Read the model definition and answer for the solid it produces. Units are mm, in the model's axes. A direction names the side the tool comes from. Give positions to 0.01 mm unless a question says otherwise; leave off trailing zeros. Order: outer loops, then holes, each group sorted by start corner. A loop starts at its lowest first (then second) coordinate and runs counter-clockwise, first axis right, second up.
Item 1: Which of the six approach directions +Z, -Z, +X, -X, +Y, -Y give full straight-line access (tool end or side, diameter ignored) to faces 5 (the face through (20, 21, -20)), 6 (the face through (35, 0, -20)), 7 (the face through (58, 21, -30))?
Item 2: The mould has two halves that part along X. Classify faces 1 (the face through (20, 30, -30)), 2 (the face through (0, 15, -25)), 3 (the face through (70, 5, -20)), 4 (the face through (5, 40, -30)): +X half, -X half, draft (parallel to the pull), parting line (faces both ways), or undercut.
Item 3: A cutting plane is placed at C-C (x = 20). Write down the section's boundary in (y, z), plus the area to 3 significant figures.
Item 4: Given pin 1 Ø6 at (x, y) = (44, 25.5) entering from +Z; pin 2 Ø16 at (x, y) = (61, 21.5) entering from +Z; pin 3 Ø9 at (x, y) = (22.5, 21.5) entering from +Z; pin 4 Ø3 at (y, z) = (27.5, -18) entering from -X, each flat-ended and moving along its own axis, determine where each tip first touches the part or whether it passes through.
Item 5: A cutting plane is placed at D-D (x = 61). Write down the section's boundary in (y, z).
Item 6: A cutting plane is placed at B-B (z = -36.5). Write down the section's boundary in (x, y), plus the area to 3 significant figures.
Item 7: Find the intervals of material crossed by line 1 along Z through (x, y) = (60, 11); line 2 along Y through (x, z) = (18, -14); line 3 along Z through (x, y) = (12, 17.5), in increasing order.
Autodesk Inventor part; units mm, degrees
ref_plane "YZ Plane" through (0, 0, 0) normal (1, 0, 0) x (0, 1, 0)
ref_plane "XZ Plane" through (0, 0, 0) normal (0, 1, 0) x (-1, 0, 0)
ref_plane "XY Plane" through (0, 0, 0) normal (0, 0, 1) x (1, 0, 0)
sketch "草圖1" plane through (0, 0, 0) normal (0, 1, 0) x (-1, 0, 0)
  line L0 (0, 0) -> (-70, 0)
  line L1 (-70, 0) -> (-70, -40)
  line L2 (-70, -40) -> (0, -40)
  line L3 (0, -40) -> (0, 0)
  dimension "d0" = 40
  dimension "d1" = 70
extrude "擠出1" add sketch "草圖1" along normal blind 10
sketch "草圖2" plane through (0, 10, 0) normal (0, 1, 0) x (1, 0, 0)
  line L0 (0, 40) -> (0, 0)
  line L1 (0, 40) -> (40, 40)
  line L2 (40, 40) -> (40, 20)
  line L3 (40, 20) -> (0, 20)
  line L4 (0, 20) -> (0, 40)
  line L5 (40, 40) -> (70, 40)
  line L6 (70, 40) -> (70, 30)
  line L7 (70, 30) -> (40, 30)
  line L8 (40, 30) -> (40, 40)
  dimension "d4" = 30
  dimension "d5" = 40
  dimension "d6" = 20
  dimension "d7" = 10
extrude "擠出2" add sketch "草圖2" along normal blind 30
chamfer "倒角1" distance 10 angle 45 1 edges at (40, 25, -30)
chamfer "倒角2" distance 20 distance2 30 1 edges at (70, 40, -35) measured on face at (13.3333, 40, -26.6668)
sketch "草圖3" plane through (0, 10, -20) normal (0, 0, 1) x (1, 0, 0)
  line L0 (0, 30) -> (40, 30)
  circle A0 centre (20, 30) radius 10
  point P0 (0, -10)
  dimension "d16" = 20
extrude "擠出3" cut sketch "草圖3" against normal blind 30
properties part number "28"
Response values:
1. face 5: +Z, +X, -X, +Y
1. face 6: +Z, -Z, +X, -X, -Y
1. face 7: +Z, +X, +Y
2. face 1: undercut
2. face 2: -X half
2. face 3: +X half
2. face 4: draft
3. outline: (0, -40) - (30, -40) - (30, -20) - (10, -20) - (10, 0) - (0, 0) - close
3. area: 800 mm2
4. pin 1: stops at z = -21
4. pin 2: stops at z = -30
4. pin 3: stops at z = -20
4. pin 4: passes through
5. outline: (0, -40) - (23.5, -40) - (23.5, -30) - (10, -30) - (10, 0) - (0, 0) - close
6. outline: (0, 0) - (70, 0) - (70, 10) - (50, 40) - (30, 40) arc R10 cw to (10, 40) - (0, 40) - close
6. area: 2,340 mm2
7. line 1: z = -40 to -30
7. line 2: y = 0 to 10
7. line 3: z = -40 to -20
